from build123d import *

# Parameters (mm, degrees)
SKETCH1_W           = 102
SKETCH1_H           = 52
SKETCH1_W_2         = 78
SKETCH1_H_2         = 31
BOSS_EXTRUDE1_DEPTH = 3
SKETCH2_R           = 2.5
CUT_EXTRUDE6_DEPTH  = 31


with BuildPart() as part:
    # Sketch1 → Boss-Extrude1 (new body)
    with BuildSketch(Plane.XY):
        Rectangle(SKETCH1_W, SKETCH1_H)
        Rectangle(SKETCH1_W_2, SKETCH1_H_2, mode=Mode.SUBTRACT)
    extrude(amount=BOSS_EXTRUDE1_DEPTH)

    # Sketch2 → Cut-Extrude6 (cut)
    with BuildSketch(Plane.XY):
        with Locations(Location((-45, 20, 0), (0, 0, 180))):
            Circle(SKETCH2_R)
        with Locations(Location((-45, -20, 0), (0, 0, 180))):
            Circle(SKETCH2_R)
        with Locations(Location((45, -20, 0), (0, 0, 180))):
            Circle(SKETCH2_R)
        with Locations(Location((45, 20, 0), (0, 0, 180))):
            Circle(SKETCH2_R)
    extrude(amount=CUT_EXTRUDE6_DEPTH, mode=Mode.SUBTRACT)


solid = part.part
Geometry: final body of the model. Coordinates: model frame, mm. A direction names the side the tool comes from. Coordinates: 2 decimals unless noted, no trailing zeros. Loops run counter-clockwise (first coordinate to the right, second up) from the corner with the lowest first, then second, coordinate; pieces in that order, holes last. Notation, with made-up numbers: (-4.75, 57.5) - (8.25, 57.5) arc R14 ccw to (8.25, 76.5) - close; hole circle Ø10 at (-26, -33). An arc over 180 degrees is marked (long way). One line per question, with ' | ' between items. Start each with the question number.
(1) Cut plane D-D on x = -45. Output: boundary loops of the cut face in (y, z).
(2) Draft query along Y for faces 1 (the flat face through (-1, -26, 1)), 2 (the flat face through (-1, 15.5, 1)), 3 (the flat face through (-1, 26, 1)), 4 (the flat face through (-1, -17, 0)). Return one class per face: +Y half, -Y half, draft (parallel to the pull), parting line (faces both ways), or undercut.
(3) Cut plane A-A on y = 20. Output: boundary loops of the cut face in (x, z).
(4) Cut plane C-C on y = 7.5. Output: boundary loops of the cut face in (x, z).
(5) Cut plane B-B on z = 2.15. Output: boundary loops of the cut face in (x, y), and give its area (3 significant figures).
(6) Reachability of faces 5 (the flat face through (51, 0, 1)), 6 (the flat face through (-1, -15.5, 1)) from +Z, -Z, +X, -X, +Y, -Y: full face, straight path, thin tool, end or side. Return the list, or none.
(7) Ray query, L1, parallel to X at y = 20, z = 2; L2, parallel to Y at x = -45, z = 2; L3, parallel to Y at x = 26.5, z = 0.4. Return the intervals inside material, ascending. Write a range as from..to.
Here are the results:
1) outline: (-26, 0) - (-22.5, 0) - (-22.5, 3) - (-26, 3) - close; (-17.5, 0) - (17.5, 0) - (17.5, 3) - (-17.5, 3) - close; (22.5, 0) - (26, 0) - (26, 3) - (22.5, 3) - close
2) face 1: -Y half | face 2: undercut | face 3: +Y half | face 4: draft
3) outline: (-51, 0) - (-47.5, 0) - (-47.5, 3) - (-51, 3) - close; (-42.5, 0) - (42.5, 0) - (42.5, 3) - (-42.5, 3) - close; (47.5, 0) - (51, 0) - (51, 3) - (47.5, 3) - close
4) outline: (-51, 0) - (-39, 0) - (-39, 3) - (-51, 3) - close; (39, 0) - (51, 0) - (51, 3) - (39, 3) - close
5) outline: (-51, -26) - (51, -26) - (51, 26) - (-51, 26) - close; hole circle Ø5 at (-45, -20); hole circle Ø5 at (-45, 20); hole (-39, -15.5) - (39, -15.5) - (39, 15.5) - (-39, 15.5) - close; hole circle Ø5 at (45, -20); hole circle Ø5 at (45, 20) | area: 2,810 mm²
6) face 5: +Z, -Z, +X, +Y, -Y | face 6: +Z, -Z
7) L1: -51..-47.5, -42.5..42.5, 47.5..51 | L2: -26..-22.5, -17.5..17.5, 22.5..26 | L3: -26..-15.5, 15.5..26
